Check sheet for the modelled part. Datum: model origin and axes. Units: mm. A direction names the side the tool comes from. Round coordinates to 2 decimals unless told otherwise and drop trailing zeros. Write each loop counter-clockwise with the first axis right and the second up, starting at its lowest first coordinate (ties: lowest second). Pieces come first, ordered by that corner, then holes.
from build123d import *

# Parameters (mm, degrees)
F0_W     = 30
F0_H     = 30
F1_DEPTH = 30
F2_R     = 5
F3_DEPTH = 30
F4_R     = 2.5
F5_DEPTH = 60.001
F6_R     = 5


with BuildPart() as f1:
    # F0 (on Front) → F1 (new body)
    with BuildSketch(Plane.XZ):
        Rectangle(F0_W, F0_H)
    extrude(amount=-F1_DEPTH)

    # F2 (on face) → F3 (join)
    with BuildSketch(Plane.XZ):
        Circle(F2_R)
    extrude(amount=F3_DEPTH)

    # F4 (on face) → F5 (cut, through all)
    with BuildSketch(Plane.XZ.offset(30)):
        Circle(F4_R)
    extrude(amount=-F5_DEPTH, mode=Mode.SUBTRACT)

    # F6
    f6_edges = [f1.edges().sort_by_distance(p)[0] for p in [
        (-15, 0, 0),
        (0, 0, -15),
        (0, 0, 15),
        (15, 0, 0),
        (-15, 15, 15),
        (15, 15, 15),
        (0, 30, 15),
        (-15, 30, 0),
        (-15, 15, -15),
        (0, 30, -15),
        (15, 15, -15),
    ]]
    fillet(f6_edges, radius=F6_R)


solid = f1.part
1. Release check for a two-part mould opening along X. For faces 3 (the flat face through (0, 15, 15)), 4 (the cylindrical face through (13, 1, 0)), 5 (the cylindrical face through (-0.54, -0.42, -2.44)) record: released by +X, released by -X, zero draft, split by the parting line, or undercut.
2. Sectioned sample at B-B, the plane x = 0. Enter the section's corners in (y, z).
3. Sectioned sample at D-D, the plane x = -9. Enter the section's corners in (y, z), plus the area to 3 significant figures.
4. Scan lines: line 1 along Z through (x, y) = (0, -10); line 2 along Z through (x, y) = (0, 10); line 3 along Y through (x, z) = (8.5, -3.25). Record each from-to range of solid material in increasing order.
5. Sectioned sample at C-C, the plane y = 22.5. Enter the section's corners in (x, z), plus the area to 3 significant figures.
6. Sectioned sample at A-A, the plane z = 0. Enter the section's corners in (x, y).
7. Set-up check for faces 1 (the cylindrical face through (0, 2, -14)), 2 (the flat face through (-2, 0, 5)): record each of +Z, -Z, +X, -X, +Y, -Y from which the full face is reachable in a straight line by a thin tool's end or side.
8. Go/stop test with flat-tipped pins: pin 1 (3 mm diameter, centred on x = -6.5, z = 10.5, fed in from -Y); pin 2 (5 mm diameter, centred on y = 1.5, z = -7.5, fed in from -X); pin 3 (4 mm diameter, centred on x = 0, z = 0, fed in from +Y). Record where each tip stops, or that it passes through.
Computed values:
1. face 3: zero draft
1. face 4: released by +X
1. face 5: undercut
2. outline: (-30, -5) - (0, -5) - (0, -10) arc R5 ccw to (5, -15) - (25, -15) arc R5 ccw to (30, -10) - (30, -2.5) - (-30, -2.5) - close; (-30, 2.5) - (30, 2.5) - (30, 10) arc R5 ccw to (25, 15) - (5, 15) arc R5 ccw to (0, 10) - (0, 5) - (-30, 5) - close
3. outline: (0, -10) arc R5 ccw to (5, -15) - (25, -15) arc R5 ccw to (30, -10) - (30, 10) arc R5 ccw to (25, 15) - (5, 15) arc R5 ccw to (0, 10) - close
3. area: 879 mm2
4. line 1: z = -5 to -2.5, 2.5 to 5
4. line 2: z = -15 to -2.5, 2.5 to 15
4. line 3: y = 0 to 30
5. outline: (-15, -10) arc R5 ccw to (-10, -15) - (10, -15) arc R5 ccw to (15, -10) - (15, 10) arc R5 ccw to (10, 15) - (-10, 15) arc R5 ccw to (-15, 10) - close; hole circle Ø5 at (0, 0)
5. area: 859 mm2
6. outline: (-15, 5) arc R5 ccw to (-10, 0) - (-5, 0) - (-5, -30) - (-2.5, -30) - (-2.5, 30) - (-10, 30) arc R5 ccw to (-15, 25) - close; (2.5, -30) - (5, -30) - (5, 0) - (10, 0) arc R5 ccw to (15, 5) - (15, 30) - (2.5, 30) - close
7. face 1: -Z, +X, -X, -Y
7. face 2: -Y
8. pin 1: stops at y = 0
8. pin 2: stops at x = -14.9
8. pin 3: passes through
